```python
from build123d import *

# Parameters (mm, degrees)
SKETCH2_R           = 15
BOSS_EXTRUDE1_DEPTH = 39


with BuildPart() as part:
    # Sketch2 → Boss-Extrude1 (new body)
    with BuildSketch(Plane.XY):
        with BuildLine():
            Line((0, 0), (-127.68773646, 0))
            Line((-127.68773646, 0), (-127.68773646, 17.025031528))
            Line((-127.68773646, 17.025031528), (-97.893931286, 17.025031528))
            Line((-97.893931286, 17.025031528), (-97.893931286, 12.768773646))
            Line((-97.893931286, 12.768773646), (-76.612641876, 12.768773646))
            Line((-76.612641876, 12.768773646), (-76.612641876, 17.025031528))
            Line((-76.612641876, 17.025031528), (-51.075094584, 17.025031528))
            Line((-51.075094584, 17.025031528), (-51.075094584, 34.050063056))
            ThreePointArc((-51.075094584, 34.050063056), (-25.537547292, 59.587610348), (0, 34.050063056))
            Line((0, 34.050063056), (0, 0))
        make_face()
        with Locations((-25.537547292, 34.050063056)):
            Circle(SKETCH2_R, mode=Mode.SUBTRACT)
    extrude(amount=BOSS_EXTRUDE1_DEPTH)


solid = part.part
```
Here's how the part is built. I have some questions about the finished solid (model axes, mm). A direction names the side the tool comes from. Coordinates: 2 decimals unless noted, no trailing zeros. Loops run counter-clockwise (first coordinate to the right, second up) from the corner with the lowest first, then second, coordinate; pieces in that order, holes last. Notation, with made-up numbers: (-3, 13) - (27, 13) arc R24 cw to (27, 38) - close; hole circle Ø6 at (-37, -27.5). An arc over 180 degrees is marked (long way). Return JSON: item names as keys, results as strings. Group by question number.
Item 1: On a 3-axis mill with a long thin cutter (end or side, diameter ignored), from which of +Z, -Z, +X, -X, +Y, -Y can I reach the whole of each face in a straight line? I mean faces 1 (the face through (-49, 24, 0)), 2 (the face through (-113, 17.025, 19)), 3 (the face through (-97.894, 15, 19)). Say none if no direction works.
Item 2: Will these pins go through, and if not, where does the flat tip stop? P1, Ø7.5, axis at x = -59, z = 18.5, coming from the +Y side; P2, Ø24, axis at x = -25.54, y = 34.05, coming from the -Z side; P3, Ø1.3, axis at y = 15, z = 19.5, coming from the +X side; P4, Ø18.5, axis at y = 29, z = 26, coming from the -X side.
Item 3: If we section it at A-A on x = -24: Write out the boundary of the cut face in (y, z).
Item 4: If we section it at D-D on x = -62.5: Write out the boundary of the cut face in (y, z), and give its area (3 significant figures).
Item 5: I need wall thicknesses on line 1 (X direction, y = 14.5, z = 2.5); line 2 (X direction, y = 34.5, z = 6); line 3 (Y direction, x = -120, z = 34). Which ranges of each line are inside material? Lowest first, please. Write a range as from..to.
Item 6: We'd pull the mould along X, two halves only. Please class faces 4 (the face through (-127.688, 8, 19)), 5 (the face through (-63, 0, 19)), 6 (the face through (-36.59, 44.19, 19.23)): +X half, -X half, draft (parallel to the pull), parting line (faces both ways), or undercut.
Item 7: If we section it at C-C on z = 18.5: Write out the boundary of the cut face in (x, y), and give its area (3 significant figures).
Item 8: If we section it at B-B on y = 21: Write out the boundary of the cut face in (x, z).
Calculated:
{
 "1": {"face 1": "-Z, +X, -X, +Y, -Y", "face 2": "+Z, -Z, -X, +Y", "face 3": "+Z, -Z, +Y"},
 "2": {"P1": "stops at y = 17.03", "P2": "passes through", "P3": "stops at x = 0", "P4": "stops at x = -51.08"},
 "3": {"outline": "(0, 0) - (19.13, 0) - (19.13, 39) - (0, 39) - close; (48.97, 0) - (59.54, 0) - (59.54, 39) - (48.97, 39) - close"},
 "4": {"outline": "(0, 0) - (17.03, 0) - (17.03, 39) - (0, 39) - close", "area": "664 mm^2"},
 "5": {"line 1": "x = -127.69..-97.89, -76.61..0", "line 2": "x = -51.07..-40.53, -10.54..0", "line 3": "y = 0..17.03"},
 "6": {"face 4": "-X half", "face 5": "draft", "face 6": "undercut"},
 "7": {"outline": "(-127.69, 0) - (0, 0) - (0, 34.05) arc R25.54 ccw to (-51.08, 34.05) - (-51.08, 17.03) - (-76.61, 17.03) - (-76.61, 12.77) - (-97.89, 12.77) - (-97.89, 17.03) - (-127.69, 17.03) - close; hole circle Ø30 at (-25.54, 34.05)", "area": "3,270 mm^2"},
 "8": {"outline": "(-51.08, 0) - (-32.93, 0) - (-32.93, 39) - (-51.08, 39) - close; (-18.14, 0) - (0, 0) - (0, 39) - (-18.14, 39) - close"}
}
